```python
from build123d import *

# Parameters (mm, degrees)
PAD006_DEPTH    = 550
SKETCH015_W     = 227
SKETCH015_H     = 96
POCKET008_DEPTH = 85
SKETCH016_W     = 37
SKETCH016_H     = 140
POCKET009_DEPTH = 65
SKETCH019_W     = 12.5
SKETCH019_H     = 21
POCKET014_DEPTH = 245.001
FILLET_R        = 5
CHAMFER_SIZE    = 3


with BuildPart() as part:
    # Sketch014 → Pad006 (new body)
    with BuildSketch(Plane.XZ):
        Polygon((0, 245), (0, 0), (-65, -24), (-65, -80), (133, -80), (133, 245), align=None)
    extrude(amount=PAD006_DEPTH)

    # Sketch015 (on Face1 of Pad006) → Pocket008 (cut)
    with BuildSketch(Plane(origin=(0, 0, 0), x_dir=(0, 0, -1), z_dir=(-1, 0, 0))):
        with Locations((-121.5, 52)):
            Rectangle(SKETCH015_W, SKETCH015_H)
        with Locations((-121.5, 198)):
            Rectangle(SKETCH015_W, SKETCH015_H)
        with Locations((-121.5, 344)):
            Rectangle(SKETCH015_W, SKETCH015_H)
        with Locations((-121.5, 490)):
            Rectangle(SKETCH015_W, SKETCH015_H)
    extrude(amount=-POCKET008_DEPTH, mode=Mode.SUBTRACT)

    # Sketch016 → Pocket009 (cut, symmetric)
    with BuildSketch(Plane.YZ):
        with Locations((-50.5, 5)):
            Rectangle(SKETCH016_W, SKETCH016_H)
        with Locations((-199.911025, 5)):
            Rectangle(SKETCH016_W, SKETCH016_H)
        with Locations((-344.615598, 5)):
            Rectangle(SKETCH016_W, SKETCH016_H)
        with Locations((-492.327623, 5)):
            Rectangle(SKETCH016_W, SKETCH016_H)
    extrude(amount=POCKET009_DEPTH, both=True, mode=Mode.SUBTRACT)

    # Sketch019 → Pocket014 (cut, through all)
    with BuildSketch(Plane.XY):
        with Locations((6.25, -33)):
            Rectangle(SKETCH019_W, SKETCH019_H)
        with Locations((6.25, -67)):
            Rectangle(SKETCH019_W, SKETCH019_H)
        with Locations((6.25, -183)):
            Rectangle(SKETCH019_W, SKETCH019_H)
        with Locations((6.25, -217)):
            Rectangle(SKETCH019_W, SKETCH019_H)
        with Locations((6.25, -328)):
            Rectangle(SKETCH019_W, SKETCH019_H)
        with Locations((6.25, -362)):
            Rectangle(SKETCH019_W, SKETCH019_H)
        with Locations((6.25, -476)):
            Rectangle(SKETCH019_W, SKETCH019_H)
        with Locations((6.25, -510)):
            Rectangle(SKETCH019_W, SKETCH019_H)
    extrude(amount=POCKET014_DEPTH, mode=Mode.SUBTRACT)

    # Fillet
    fillet_edges = [part.edges().sort_by_distance(p)[0] for p in [
        (-65, -16, -24),
        (-65, -125.205513, -24),
        (-65, -272.263312, -24),
        (-65, -418.47161, -24),
        (-65, -530.413811, -24),
    ]]
    fillet(fillet_edges, radius=FILLET_R)

    # Chamfer
    chamfer_edges = [part.edges().sort_by_distance(p)[0] for p in [
        (0, -100, 121.5),
        (0, -150, 121.5),
        (0, -246, 121.5),
        (0, -296, 121.5),
        (0, -392, 121.5),
        (0, -442, 121.5),
        (0, -538, 121.5),
        (0, -4, 121.5),
    ]]
    chamfer(chamfer_edges, length=CHAMFER_SIZE)


with BuildPart() as part_1:
    # Body004 placement: moved
    add(part.part.moved(Location((0, 43, 0))))


solid = part_1.part
```
The listing builds one solid part. Answer for the finished solid, in the listing's coordinates (mm). A direction names the side the tool comes from. Give positions to 0.01 mm unless a question says otherwise; leave off trailing zeros. Order: outer loops, then holes, each group sorted by start corner. A loop starts at its lowest first (then second) coordinate and runs counter-clockwise, first axis right, second up. Notation, with made-up numbers: (0.5, -29) -> (49.5, -29) arc R13 cw to (49.5, -11) -> close; hole circle Ø8 at (-14.75, 0). An arc over 180 degrees is marked (long way). Answer as a JSON object with one key per item and string values. Group by question number.
Item 1: A tool of negligible diameter and unlimited length cuts with its end or side. For faces 3 (the flat face through (0, -375, 124)), 4 (the flat face through (85, -156, 123)), 5 (the flat face through (-65, -228, -53)), from which of +Z, -Z, +X, -X, +Y, -Y can it reach the whole face along a straight path? Write none if from no direction.
Item 2: Flat-ended cylindrical pins translate along their axes: pin 1 (11 mm diameter, centred on y = 29.5, z = 132.5, fed in from -X); pin 2 (18.5 mm diameter, centred on y = -165.5, z = -38.5, fed in from -X); pin 3 (5 mm diameter, centred on y = -318, z = 240, fed in from -X). Find the tip coordinate at first contact, or state that the pin passes through.
Item 3: Consider L1, parallel to Y at x = 20, z = 27.5; L2, parallel to Y at x = 55, z = -34; L3, parallel to Z at x = 69, y = -144.5. Determine where each line is inside the solid, lowest interval first. Write a range as from..to.
Item 4: The part is cut by section D-D on y = -289.5. Write down the section's boundary in (x, z).
Item 5: Determine the mould class of faces 1 (the flat face through (33, -228, -80)), 2 (the flat face through (-1, -302, -65)) for opening direction Y: pulls with the +Y half, pulls with the -Y half, needs draft (parallel to the pull), parting line crosses it, or undercut.
Item 6: The part is cut by section A-A on y = -122. Write down the section's boundary in (x, z), and give its area (3 significant figures).
Item 7: The part is cut by section B-B on z = -48. Write down the section's boundary in (x, y).
Item 8: The part is cut by section C-C on x = -37.5. Write down the section's boundary in (y, z), and give its area (3 significant figures).
Result set:
{
 "1": {"face 3": "+Z, -X, +Y, -Y", "face 4": "-X", "face 5": "+Z, -Z, -X, +Y, -Y"},
 "2": {"pin 1": "x = 85", "pin 2": "x = 65", "pin 3": "x = 12.5"},
 "3": {"L1": "-507..-495, -399..-349, -253..-203, -107..-57, 39..43", "L2": "-507..-467.83, -430.83..-320.12, -283.12..-175.41, -138.41..-26, 11..43", "L3": "-80..8, 235..245"},
 "4": {"outline": "(-65, -80) -> (133, -80) -> (133, 245) -> (12.5, 245) -> (12.5, 235) -> (85, 235) -> (85, 8) -> (65, 8) -> (65, -65) -> (-65, -65) -> close"},
 "5": {"face 1": "needs draft", "face 2": "undercut"},
 "6": {"outline": "(-65, -80) -> (133, -80) -> (133, 245) -> (0, 245) -> (0, 235) -> (85, 235) -> (85, 8) -> (0, 8) -> (0, 0) -> (-61.73, -22.79) arc R5 ccw to (-65, -27.48) -> close", "area": "28,300 mm²"},
 "7": {"outline": "(-65, -507) -> (133, -507) -> (133, 43) -> (-65, 43) -> (-65, 11) -> (65, 11) -> (65, -26) -> (-65, -26) -> (-65, -138.41) -> (65, -138.41) -> (65, -175.41) -> (-65, -175.41) -> (-65, -283.12) -> (65, -283.12) -> (65, -320.12) -> (-65, -320.12) -> (-65, -430.83) -> (65, -430.83) -> (65, -467.83) -> (-65, -467.83) -> close"},
 "8": {"outline": "(-507, -80) -> (43, -80) -> (43, -13.85) -> (11, -13.85) -> (11, -65) -> (-26, -65) -> (-26, -13.85) -> (-138.41, -13.85) -> (-138.41, -65) -> (-175.41, -65) -> (-175.41, -13.85) -> (-283.12, -13.85) -> (-283.12, -65) -> (-320.12, -65) -> (-320.12, -13.85) -> (-430.83, -13.85) -> (-430.83, -65) -> (-467.83, -65) -> (-467.83, -13.85) -> (-507, -13.85) -> close", "area": "28,800 mm²"}
}
